CAD build for the part. Positions are in the model's coordinates, mm. Give positions to 0.01 mm unless a question says otherwise; leave off trailing zeros. Order: outer loops, then holes, each group sorted by start corner. A loop starts at its lowest first (then second) coordinate and runs counter-clockwise, first axis right, second up. Notation, with made-up numbers: (-26, -35.5) -> (-21, -35.5) arc R10 cw to (-21, -19.5) -> close; hole circle Ø1 at (6, -35). An arc over 180 degrees is marked (long way). Use one line per item in the form item = value. Start each with the question number.
1) Cut at B-B, the plane z = 2.05. Give the cut face in (x, y), and give its area (3 significant figures).
2) Cut at C-C, the plane y = -241. Give the cut face in (x, z), and give its area (3 significant figures).
3) Drop flat-ended pins along their axis: P1, Ø1.5, axis at x = -303, z = 3, coming from the +Y side; P2, Ø2.5, axis at y = -267.5, z = 3.5, coming from the +X side; P3, Ø6, axis at x = -203.5, y = -230, coming from the -Z side; P4, Ø2.5, axis at x = -303, z = 3.5, coming from the -Y side. Give the stop position or say it passes through.
4) Probe line 1 (X direction, y = -24, z = 3); line 2 (X direction, y = -280, z = 2.3); line 3 (X direction, y = -23.5, z = 1.15). List the from-to ranges inside material, lowest first.
5) Cut at A-A, the plane x = -139.5. Give the cut face in (y, z).
from build123d import *

# Parameters (mm, degrees)
ESQUISSE1_W                        = 300
ESQUISSE1_H                        = 295
BOSS_EXTRU_1_DEPTH                 = 5
TENON_START                        = -182
TENON_ET_MORTAISE_TENON1_OUTLINE_W = 5
TENON_ET_MORTAISE_TENON1_OUTLINE_H = 5
TENON_ET_MORTAISE_TENON1_DEPTH     = 72
TENON_ET_MORTAISE_TENON2_OUTLINE_W = 5
TENON_ET_MORTAISE_TENON2_OUTLINE_H = 5
TENON_ET_MORTAISE_TENON2_DEPTH     = 72
ESQUISSE2_W                        = 59.408594242
ESQUISSE2_H                        = 27.612445211
ENL_V_MAT_EXTRU_2_DEPTH            = 10
ESQUISSE3_R                        = 2.100000001
ENL_V_MAT_EXTRU_3_DEPTH            = 425.352447854
ESQUISSE4_R                        = 2.1
ENL_V_MAT_EXTRU_4_DEPTH            = 425.352447854
ESQUISSE5_R                        = 2.1
ENL_V_MAT_EXTRU_5_DEPTH            = 425.352447854


# Read off the part's stored shape, not the designer's step: Tenon et mortaise-Tenon1, Tenon et mortaise-Tenon2
with BuildPart() as part:
    # Esquisse1 → Boss.-Extru.1 (new body)
    with BuildSketch(Plane.XY):
        with Locations((-150, -147.5)):
            Rectangle(ESQUISSE1_W, ESQUISSE1_H)
    extrude(amount=BOSS_EXTRU_1_DEPTH)

    # Tenon et mortaise-Tenon1 outline → Tenon et mortaise-Tenon1 (add)
    with BuildSketch(Plane(origin=(0, 0, 0), x_dir=(1, 0, 0), z_dir=(0, 1, 0)).offset(TENON_START)):
        with Locations((2.5, -2.5)):
            Rectangle(TENON_ET_MORTAISE_TENON1_OUTLINE_W, TENON_ET_MORTAISE_TENON1_OUTLINE_H)
    extrude(amount=TENON_ET_MORTAISE_TENON1_DEPTH)

    # Tenon et mortaise-Tenon2 outline → Tenon et mortaise-Tenon2 (add)
    with BuildSketch(Plane(origin=(0, 0, 0), x_dir=(1, 0, 0), z_dir=(0, 1, 0)).offset(TENON_START)):
        with Locations((-302.5, -2.5)):
            Rectangle(TENON_ET_MORTAISE_TENON2_OUTLINE_W, TENON_ET_MORTAISE_TENON2_OUTLINE_H)
    extrude(amount=TENON_ET_MORTAISE_TENON2_DEPTH)

    # Esquisse2 → Enlèv. mat.-Extru.2 (cut)
    with BuildSketch(Plane(origin=(0, 0, 0), x_dir=(-1, 0, 0), z_dir=(0, 0, -1))):
        with Locations((153.346963056, -267.352892149)):
            Rectangle(ESQUISSE2_W, ESQUISSE2_H)
    extrude(amount=-ENL_V_MAT_EXTRU_2_DEPTH, mode=Mode.SUBTRACT)

    # Esquisse3 → Enlèv. mat.-Extru.3 (cut, through all)
    with BuildSketch(Plane(origin=(0, 0, 0), x_dir=(-1, 0, 0), z_dir=(0, 0, -1))):
        with Locations((291.051040249, -219.502837044)):
            Circle(ESQUISSE3_R)
        with Locations(Location((8.948959751, -219.502837044, 0), (0, 0, 180))):
            Circle(ESQUISSE3_R)
    extrude(amount=-ENL_V_MAT_EXTRU_3_DEPTH, mode=Mode.SUBTRACT)

    # Esquisse4 → Enlèv. mat.-Extru.4 (cut, through all)
    with BuildSketch(Plane(origin=(0, 0, 0), x_dir=(-1, 0, 0), z_dir=(0, 0, -1))):
        with Locations((291.051040249, -24.502837044)):
            Circle(ESQUISSE4_R)
    extrude(amount=-ENL_V_MAT_EXTRU_4_DEPTH, mode=Mode.SUBTRACT)

    # Esquisse5 → Enlèv. mat.-Extru.5 (cut, through all)
    with BuildSketch(Plane(origin=(0, 0, 0), x_dir=(-1, 0, 0), z_dir=(0, 0, -1))):
        with Locations((291.051040249, -24.502837044)):
            Circle(ESQUISSE5_R)
        with Locations(Location((8.948959751, -24.502837044, 0), (0, 0, 180))):
            Circle(ESQUISSE5_R)
    extrude(amount=-ENL_V_MAT_EXTRU_5_DEPTH, mode=Mode.SUBTRACT)


solid = part.part
Result:
q1.outline = (-305, -182) -> (-300, -182) -> (-300, -295) -> (0, -295) -> (0, -182) -> (5, -182) -> (5, -110) -> (0, -110) -> (0, 0) -> (-300, 0) -> (-300, -110) -> (-305, -110) -> close; hole circle Ø4.2 at (-291.05, -219.5); hole circle Ø4.2 at (-291.05, -24.5); hole (-183.05, -281.16) -> (-123.64, -281.16) -> (-123.64, -253.55) -> (-183.05, -253.55) -> close; hole circle Ø4.2 at (-8.95, -219.5); hole circle Ø4.2 at (-8.95, -24.5)
q1.area = 87,500 mm²
q2.outline = (-300, 0) -> (0, 0) -> (0, 5) -> (-300, 5) -> close
q2.area = 1,500 mm²
q3.P1 = -110
q3.P2 = 0
q3.P3 = 0
q3.P4 = -182
q4.line_1 = -300 to -293.09, -289.01 to -10.99, -6.91 to 0
q4.line_2 = -300 to -183.05, -123.64 to 0
q4.line_3 = -300 to -292.9, -289.21 to -10.79, -7.1 to 0
q5.outline = (-295, 0) -> (-281.16, 0) -> (-281.16, 5) -> (-295, 5) -> close; (-253.55, 0) -> (0, 0) -> (0, 5) -> (-253.55, 5) -> close
